The model under review builds one solid part; all positions refer to its coordinate system, in mm. Face numbers are marked on the shaded views. A direction names the side the tool comes from. Give positions to 0.01 mm unless a question says otherwise; leave off trailing zeros. Loops run counter-clockwise (first coordinate to the right, second up) from the corner with the lowest first, then second, coordinate; pieces in that order, holes last. Notation, with made-up numbers: M 19,34.5 L 48,34.5 A17 ccw 48,56.5 Z; hole C 67.5,35 d1. An arc over 180 degrees is marked long. Return JSON: item names as keys, results as strings.
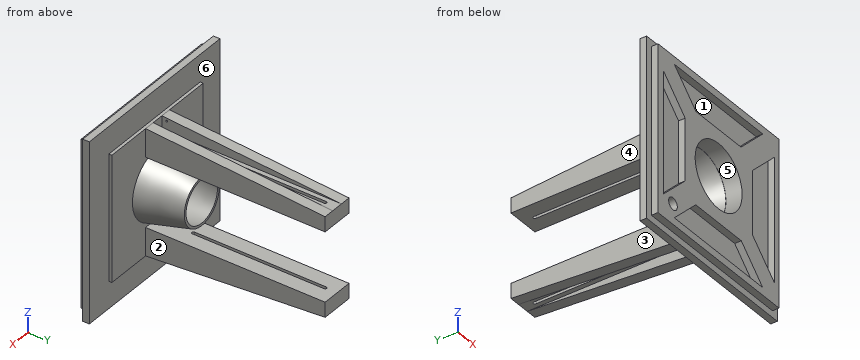
```python
from build123d import *

# Parameters (mm, degrees)
SKETCH2_W               = 210
SKETCH2_H               = 5
BOSS_EXTRUDE1_DEPTH     = 105
SKETCH5_W               = 55.001300882
SKETCH5_H               = 25
BOSS_EXTRUDE2_DEPTH     = 300
CUT_EXTRUDE3_DEPTH      = 25
CUT_EXTRUDE4_START      = -25
CUT_EXTRUDE4_DEPTH      = 25
SKETCH8_W               = 17.5
SKETCH8_H               = 22
BOSS_EXTRUDE3_DEPTH     = 300
CUT_EXTRUDE7_DEPTH      = 345.35628352
SKETCH12_R              = 1.5
CUT_EXTRUDE8_DEPTH      = 20
SKETCH13_W              = 300.5
SKETCH13_H              = 300.5
BOSS_EXTRUDE4_DEPTH     = 11
SKETCH4_R               = 54
CUT_EXTRUDE2_DEPTH      = 20
SKETCH14_W              = 278.5
SKETCH14_H              = 278.5
SKETCH14_R              = 54
BOSS_EXTRUDE5_DEPTH     = 11
CUT_EXTRUDE9_DEPTH      = 372.921362656
CUT_EXTRUDE9_DEPTH_BACK = 372.921362656
SKETCH16_R              = 10


with BuildPart() as part:
    # Sketch1 → Revolve1 (revolve)
    with BuildSketch(Plane(origin=(0, 0, 0), x_dir=(0, 0, -1), z_dir=(1, 0, 0)), mode=Mode.PRIVATE) as revolve1_sk:
        Polygon((58, -1.164167591), (40.125, 73.835832409), (36.125, 73.835832409), (54, -1.164167591), align=None)
    revolve(revolve1_sk.sketch.rotate(Axis((0, 0, 0), (0, -1, 0)), 180), axis=Axis((0, 0, 0), (0, -1, 0)))

    # Sketch2 → Boss-Extrude1 (add, symmetric)
    with BuildSketch(Plane.XY):
        with Locations((0, -2.5)):
            Rectangle(SKETCH2_W, SKETCH2_H)
    extrude(amount=BOSS_EXTRUDE1_DEPTH, both=True)

    # Sketch5 → Boss-Extrude2 (add)
    with BuildSketch(Plane(origin=(0, 0, 0), x_dir=(1, 0, 0), z_dir=(0, 1, 0))):
        with Locations((-0.000650441, 70.5)):
            Rectangle(SKETCH5_W, SKETCH5_H)
        with Locations((-0.000650441, -70.5)):
            Rectangle(SKETCH5_W, SKETCH5_H)
    extrude(amount=BOSS_EXTRUDE2_DEPTH)

    # Sketch6 → Cut-Extrude3 (cut)
    with BuildSketch(Plane.XY.offset(83)):
        with BuildLine():
            Line((-2.5, 280), (-2.5, 60))
            ThreePointArc((-2.5, 60), (0, 57.5), (2.5, 60))
            Line((2.5, 60), (2.5, 280))
            ThreePointArc((2.5, 280), (0, 282.5), (-2.5, 280))
        make_face()
    extrude(amount=-CUT_EXTRUDE3_DEPTH, mode=Mode.SUBTRACT)

    # Sketch7 → Cut-Extrude4 (cut)
    with BuildSketch(Plane(origin=(0, 0, -83), x_dir=(-1, 0, 0), z_dir=(0, 0, -1)).offset(CUT_EXTRUDE4_START)):
        with BuildLine():
            Line((-2.5, 280), (-2.5, 60))
            ThreePointArc((-2.5, 60), (0, 57.5), (2.5, 60))
            Line((2.5, 60), (2.5, 280))
            ThreePointArc((2.5, 280), (0, 282.5), (-2.5, 280))
        make_face()
    extrude(amount=CUT_EXTRUDE4_DEPTH, mode=Mode.SUBTRACT)

    # Sketch8 → Boss-Extrude3 (add)
    with BuildSketch(Plane(origin=(0, 0, 0), x_dir=(1, 0, 0), z_dir=(0, 1, 0))):
        with Locations((18.75, -94)):
            Rectangle(SKETCH8_W, SKETCH8_H)
        with Locations((-18.751300882, 94)):
            Rectangle(SKETCH8_W, SKETCH8_H)
        with Locations((-18.751300882, -94)):
            Rectangle(SKETCH8_W, SKETCH8_H)
        with Locations((18.75, 94)):
            Rectangle(SKETCH8_W, SKETCH8_H)
    extrude(amount=BOSS_EXTRUDE3_DEPTH)

    # Sketch11 → Cut-Extrude7 (cut, through all)
    with BuildSketch(Plane(origin=(27.5, 0, 0), x_dir=(0, 0, -1), z_dir=(1, 0, 0))):
        Polygon((-105, 0), (-83, 300), (-105, 300), align=None)
        Polygon((105, 300), (105, 0), (83, 300), align=None)
    extrude(amount=-CUT_EXTRUDE7_DEPTH, mode=Mode.SUBTRACT)

    # Sketch12 → Cut-Extrude8 (cut)
    with BuildSketch(Plane.ZY.offset(27.501300882)):
        with Locations((99.399906916, 8)):
            Circle(SKETCH12_R)
    extrude(amount=-CUT_EXTRUDE8_DEPTH, mode=Mode.SUBTRACT)

    # Sketch13 → Boss-Extrude4 (add)
    with BuildSketch(Plane.XZ.offset(5)):
        with Locations((-0.25, 0.25)):
            Rectangle(SKETCH13_W, SKETCH13_H)
    extrude(amount=BOSS_EXTRUDE4_DEPTH)

    # Sketch4 → Cut-Extrude2 (cut)
    with BuildSketch(Plane(origin=(0, 0, 0), x_dir=(1, 0, 0), z_dir=(0, 1, 0))):
        with Locations(Location((0, 0, 0), (0, 0, 270))):
            Circle(SKETCH4_R)
    extrude(amount=-CUT_EXTRUDE2_DEPTH, mode=Mode.SUBTRACT)

    # Sketch14 → Boss-Extrude5 (add)
    with BuildSketch(Plane.XZ.offset(16)):
        with Locations((-0.25, 0.25)):
            Rectangle(SKETCH14_W, SKETCH14_H)
        with Locations(Location((0, 0, 0), (0, 0, 90))):
            Circle(SKETCH14_R, mode=Mode.SUBTRACT)
        Polygon((-102, 127), (-52, 77), (51.5, 77), (101.5, 127), align=None, mode=Mode.SUBTRACT)
        Polygon((-127, 102), (-77, 52), (-77, -51.5), (-127, -101.5), align=None, mode=Mode.SUBTRACT)
        Polygon((-102, -126.5), (-52.613173487, -77.113173487), (52.113173487, -77.113173487), (101.5, -126.5), align=None, mode=Mode.SUBTRACT)
        Polygon((128.205701443, 103.705701443), (128.205701443, -103.205701443), (78.205701443, -53.205701443), (78.205701443, 53.705701443), align=None, mode=Mode.SUBTRACT)
    extrude(amount=BOSS_EXTRUDE5_DEPTH)

    # Sketch16 → Cut-Extrude9 (cut, two sides: drawn at the far end of the back side and taken through both)
    with BuildSketch(Plane(origin=(0, -5, 0), x_dir=(1, 0, 0), z_dir=(0, 1, 0)).offset(-CUT_EXTRUDE9_DEPTH_BACK)):
        with Locations(Location((-105, 105, 0), (0, 0, 180))):
            Circle(SKETCH16_R)
    extrude(amount=CUT_EXTRUDE9_DEPTH + CUT_EXTRUDE9_DEPTH_BACK, mode=Mode.SUBTRACT)


solid = part.part
```
1) Tool access review of the marked faces 3, 4, 5 and 6: name each direction out of +Z, -Z, +X, -X, +Y, -Y from which nothing blocks a thin tool from reaching the whole face with its end or side.
From the geometry:
{"face 3": "-Z, -X, +Y", "face 4": "+Z, -X, +Y", "face 5": "-Y", "face 6": "+Y"}
2) Insertion check: pin 1 (12.5 mm diameter, centred on y = 205, z = 76, fed in from +X); pin 2 (9 mm diameter, centred on x = -34, y = -22.5, fed in from -Z); pin 3 (8 mm diameter, centred on y = 83.5, z = -102, fed in from -X). Each pin has a flat end and moves straight along its axis. Give the tip position at first contact, or say it passes through.
From the geometry:
{"pin 1": "x = 27.5", "pin 2": "z = -139", "pin 3": "x = -27.5"}
3) The part is to be moulded in two halves that separate along Z. For the marked faces 1 and 2, say which applies: released by +Z, released by -Z, zero draft, split by the parting line, or undercut.
From the geometry:
{"face 1": "undercut", "face 2": "zero draft"}
4) Consider section A-A on y = 66. Write out the cut boundary in (x, z), then the cut area to 3 significant figures.
From the geometry:
{"outline": "C 0,0 d83.99; M -27.5,-100.16 L -10,-100.16 L -10,-83 L -2.5,-83 L -2.5,-58 L -27.5,-58 Z; M -27.5,58 L -2.5,58 L -2.5,83 L -10,83 L -10,100.16 L -27.5,100.16 Z; M 2.5,-83 L 10,-83 L 10,-100.16 L 27.5,-100.16 L 27.5,-58 L 2.5,-58 Z; M 2.5,58 L 27.5,58 L 27.5,100.16 L 10,100.16 L 10,83 L 2.5,83 Z; hole C 0,0 d75.99", "area": "4,710 mm²"}
5) Consider section C-C on y = 170. Write out the cut boundary in (x, z).
From the geometry:
{"outline": "M -27.5,-92.53 L -10,-92.53 L -10,-83 L -2.5,-83 L -2.5,-58 L -27.5,-58 Z; M -27.5,58 L -2.5,58 L -2.5,83 L -10,83 L -10,92.53 L -27.5,92.53 Z; M 2.5,-83 L 10,-83 L 10,-92.53 L 27.5,-92.53 L 27.5,-58 L 2.5,-58 Z; M 2.5,58 L 27.5,58 L 27.5,92.53 L 10,92.53 L 10,83 L 2.5,83 Z"}
6) Wall thickness on L1, parallel to Z at x = -105, y = -17; L2, parallel to Z at x = -105, y = -14.25; L3, parallel to X at y = -9, z = 0: over which ranges is each line inside the solid? List them lowest first. Write a range as from..to.
From the geometry:
{"L1": "-139..-115, -95..-79.5, 80..139.5", "L2": "-150..-115, -95..150.5", "L3": "-150.5..-54, 54..150"}
7) Consider section D-D on y = 241. Write out the cut boundary in (x, z), then the cut area to 3 significant figures.
From the geometry:
{"outline": "M -27.5,-87.33 L -10,-87.33 L -10,-83 L -2.5,-83 L -2.5,-58 L -27.5,-58 Z; M -27.5,58 L -2.5,58 L -2.5,83 L -10,83 L -10,87.33 L -27.5,87.33 Z; M 2.5,-83 L 10,-83 L 10,-87.33 L 27.5,-87.33 L 27.5,-58 L 2.5,-58 Z; M 2.5,58 L 27.5,58 L 27.5,87.33 L 10,87.33 L 10,83 L 2.5,83 Z", "area": "2,800 mm²"}
